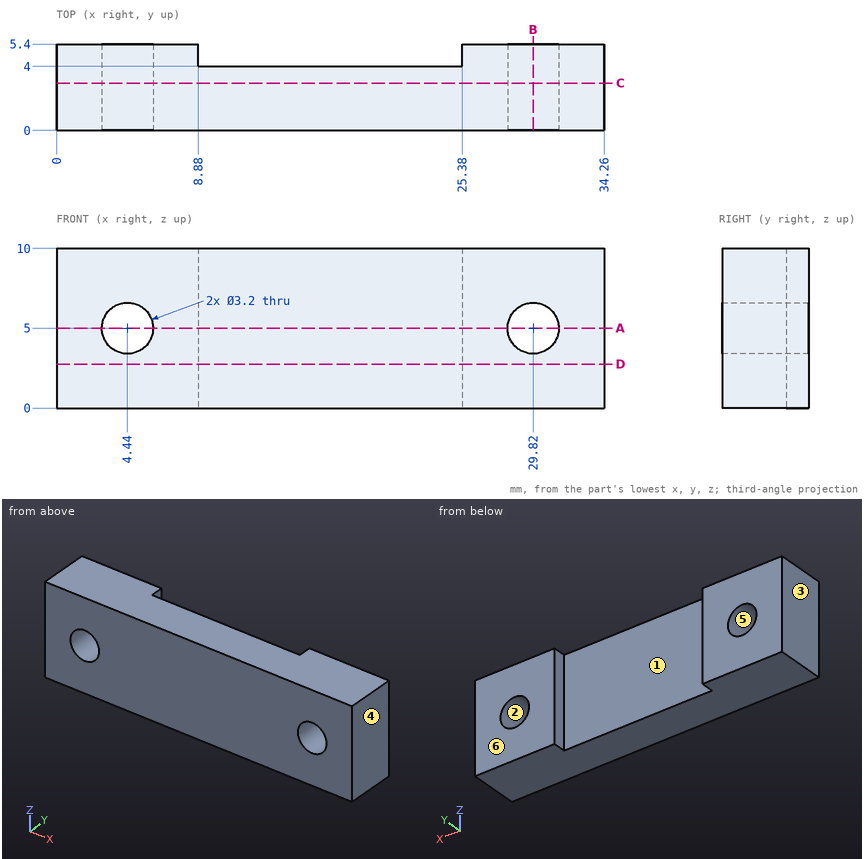
Could you check a few things on this drawing? It's one solid part, dimensions in mm from its lowest x, y, z. A direction names the side the tool comes from. Give positions to 0.01 mm unless a question says otherwise; leave off trailing zeros. Order: outer loops, then holes, each group sorted by start corner. A loop starts at its lowest first (then second) coordinate and runs counter-clockwise, first axis right, second up. Notation, with made-up numbers: (71, 54) -> (110, 54) arc R17 ccw to (110, 72) -> close; hole circle Ø10 at (85.25, 84). An arc over 180 degrees is marked (long way). Answer in a Markdown table with one row per item. Add a question column.
Item 1: Please list where these lines run through material, in increasing order: probe 1 along X at (y, z) = (4.5, 5); probe 2 along X at (y, z) = (3.55, 5); probe 3 along X at (y, z) = (4.8, 4.5).
Item 2: I'm going to push flat-ended pins straight in: P1, Ø2, axis at x = 22.5, z = 6, coming from the +Y side; P2, Ø1.9, axis at x = 29.82, z = 5, coming from the -Y side. Where does each tip first touch, or does it pass through?
Item 3: For the marked faces 1 and 2, which set-ups out of +Z, -Z, +X, -X, +Y, -Y let a thin tool reach every point of the face, with its end or its side?
Item 4: Imagine slicing it at B-B (x = 29.82). List the corners of the cut face in (y, z) for me, and give its area (3 significant figures).
Item 5: Imagine slicing it at A-A (z = 5). List the corners of the cut face in (x, y) for me, and give its area (3 significant figures).
Item 6: Imagine slicing it at C-C (y = 2.95). List the corners of the cut face in (x, z) for me.
Item 7: Imagine slicing it at D-D (z = 2.75). List the corners of the cut face in (x, y) for me.
Item 8: We'd pull the mould along X, two halves only. Please class the marked faces 3, 4, 5 and 6: pulls with the +X half, pulls with the -X half, needs draft (parallel to the pull), parting line crosses it, or undercut.
Result:
| question | item | result |
|---|---|---|
| 1 | probe 1 | 0 to 2.84, 6.04 to 8.88, 25.38 to 28.22, 31.42 to 34.26 |
| 1 | probe 2 | 0 to 2.84, 6.04 to 28.22, 31.42 to 34.26 |
| 1 | probe 3 | 0 to 2.92, 5.96 to 8.88, 25.38 to 28.3, 31.34 to 34.26 |
| 2 | P1 | y = 4 |
| 2 | P2 | through |
| 3 | face 1 | +Z, -Z, +Y |
| 3 | face 2 | +Y, -Y |
| 4 | outline | (0, 0) -> (5.4, 0) -> (5.4, 3.4) -> (0, 3.4) -> close; (0, 6.6) -> (5.4, 6.6) -> (5.4, 10) -> (0, 10) -> close |
| 4 | area | 36.7 mm2 |
| 5 | outline | (0, 0) -> (2.84, 0) -> (2.84, 5.4) -> (0, 5.4) -> close; (6.04, 0) -> (28.22, 0) -> (28.22, 5.4) -> (25.38, 5.4) -> (25.38, 4) -> (8.88, 4) -> (8.88, 5.4) -> (6.04, 5.4) -> close; (31.42, 0) -> (34.26, 0) -> (34.26, 5.4) -> (31.42, 5.4) -> close |
| 5 | area | 127 mm2 |
| 6 | outline | (0, 0) -> (34.26, 0) -> (34.26, 10) -> (0, 10) -> close; hole circle Ø3.2 at (4.44, 5); hole circle Ø3.2 at (29.82, 5) |
| 7 | outline | (0, 0) -> (34.26, 0) -> (34.26, 5.4) -> (25.38, 5.4) -> (25.38, 4) -> (8.88, 4) -> (8.88, 5.4) -> (0, 5.4) -> close |
| 8 | face 3 | pulls with the -X half |
| 8 | face 4 | pulls with the +X half |
| 8 | face 5 | undercut |
| 8 | face 6 | needs draft |
